Geometry: see drawing. Coordinates: mm, zero at the bounding-box minimum. A direction names the side the tool comes from. Give positions to 0.01 mm unless a question says otherwise; leave off trailing zeros. Write each loop counter-clockwise with the first axis right and the second up, starting at its lowest first coordinate (ties: lowest second). Pieces come first, ordered by that corner, then holes. Notation, with made-up numbers: (83.5, -18.75) - (95.5, -18.75) arc R18 ccw to (95.5, -4.75) - close; hole circle Ø1 at (3.5, 63). An arc over 180 degrees is marked (long way). Use a Markdown table: item, result. Add a question column.
1. Section query C-C, the plane z = 7.5. Return loops of the section in (x, y), plus the area to 3 significant figures.
2. Set-up query: the marked faces 1 and 2. Return all of +Z, -Z, +X, -X, +Y, -Y with unobstructed straight access to the full face (end or side cutting, diameter ignored); none if empty.
3. Section query B-B, the plane y = 457. Return loops of the section in (x, z).
4. Material intervals for probe 1 along Y at (x, z) = (457, 29.5); probe 2 along X at (y, z) = (307, 11) (1 decimal); probe 3 along X at (y, z) = (617, 22) (1 decimal), sorted ascending.
5. Section query D-D, the plane x = 663.5. Return loops of the section in (y, z) (1 decimal).
6. Pin query (flat end, axial travel): pin 1 (1 mm diameter, centred on y = 347, z = 44.5, fed in from -X); pin 2 (1 mm diameter, centred on x = 814.5, z = 24.5, fed in from +Y); pin 3 (6 mm diameter, centred on y = 652, z = 18.5, fed in from +X). Return the tip coordinate at first contact, or that it passes through.
7. Section query A-A, the plane x = 457. Return loops of the section in (y, z), plus the area to 3 significant figures.
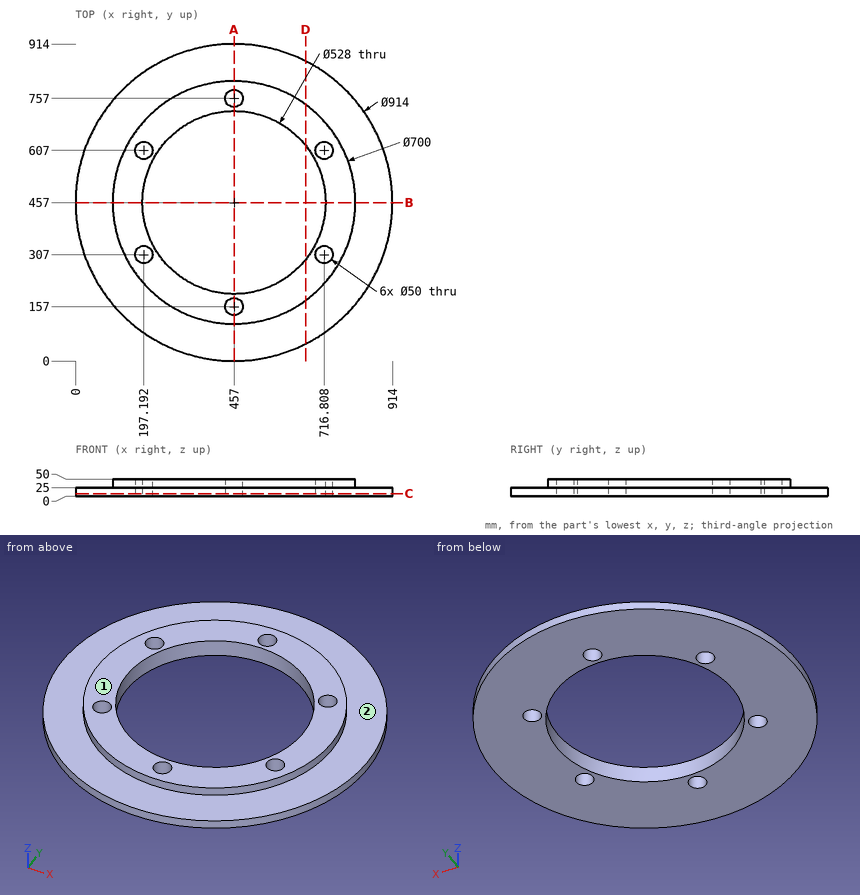
Result sheet:
| question | item | result |
|---|---|---|
| 1 | outline | circle Ø914 at (457, 457); hole circle Ø50 at (197.19, 307); hole circle Ø50 at (197.19, 607); hole circle Ø528 at (457, 457); hole circle Ø50 at (457, 157); hole circle Ø50 at (457, 757); hole circle Ø50 at (716.81, 307); hole circle Ø50 at (716.81, 607) |
| 1 | area | 425,000 mm² |
| 2 | face 1 | +Z, +X, -X, +Y, -Y |
| 2 | face 2 | +Z |
| 3 | outline | (0, 0) - (193, 0) - (193, 50) - (107, 50) - (107, 25) - (0, 25) - close; (721, 0) - (914, 0) - (914, 25) - (807, 25) - (807, 50) - (721, 50) - close |
| 4 | probe 1 | y = 107 to 132, 182 to 193, 721 to 732, 782 to 807 |
| 4 | probe 2 | x = 25.3 to 172.2, 222.2 to 239.8, 674.2 to 691.8, 741.8 to 888.7 |
| 4 | probe 3 | x = 28.9 to 174.3, 220.1 to 247, 667 to 693.9, 739.7 to 885.1 |
| 5 | outline | (49.3, 0) - (292.5, 0) - (292.5, 50) - (174.4, 50) - (174.4, 25) - (49.3, 25) - close; (621.5, 0) - (864.7, 0) - (864.7, 25) - (739.6, 25) - (739.6, 50) - (621.5, 50) - close |
| 6 | pin 1 | stops at x = 124.57 |
| 6 | pin 2 | stops at y = 742.31 |
| 6 | pin 3 | stops at x = 871.71 |
| 7 | outline | (0, 0) - (132, 0) - (132, 50) - (107, 50) - (107, 25) - (0, 25) - close; (182, 0) - (193, 0) - (193, 50) - (182, 50) - close; (721, 0) - (732, 0) - (732, 50) - (721, 50) - close; (782, 0) - (914, 0) - (914, 25) - (807, 25) - (807, 50) - (782, 50) - close |
| 7 | area | 8,950 mm² |
